Here's the drawing with two shaded views (mm, measured from the low corner). I have some questions. Give positions to 0.01 mm unless a question says otherwise; leave off trailing zeros. Loops run counter-clockwise (first coordinate to the right, second up) from the corner with the lowest first, then second, coordinate; pieces in that order, holes last. Notation, with made-up numbers: M 28.25,78 L 63.25,78 A27 cw 63.25,113 Z; hole C -5,-33 d8. An arc over 180 degrees is marked long. Put each result on its own line as item: value. Start each with the question number.
1) Imagine slicing it at A-A (z = 10). Write out the boundary of the cut face in (x, y).
2) Imagine slicing it at B-B (z = 18.25). Write out the boundary of the cut face in (x, y).
3) If we mould it in two halves opening along X, with no side actions, what happens to the marked faces 1, 2 and 3? For each: +X half, -X half, draft (parallel to the pull), parting line (faces both ways), or undercut.
4) For P1, Ø1.5, axis at x = 4.5, y = 5.5, coming from the -Z side, with a flat end and sliding along its axis, tell me the tip position at first contact or that it passes through.
5) Please list where these lines run through material, in increasing order: line 1 along Z through (x, y) = (3, 2); line 2 along X through (y, z) = (4.8, 10); line 3 along Z through (x, y) = (1.75, 4) (1 decimal). Write a range as from..to.
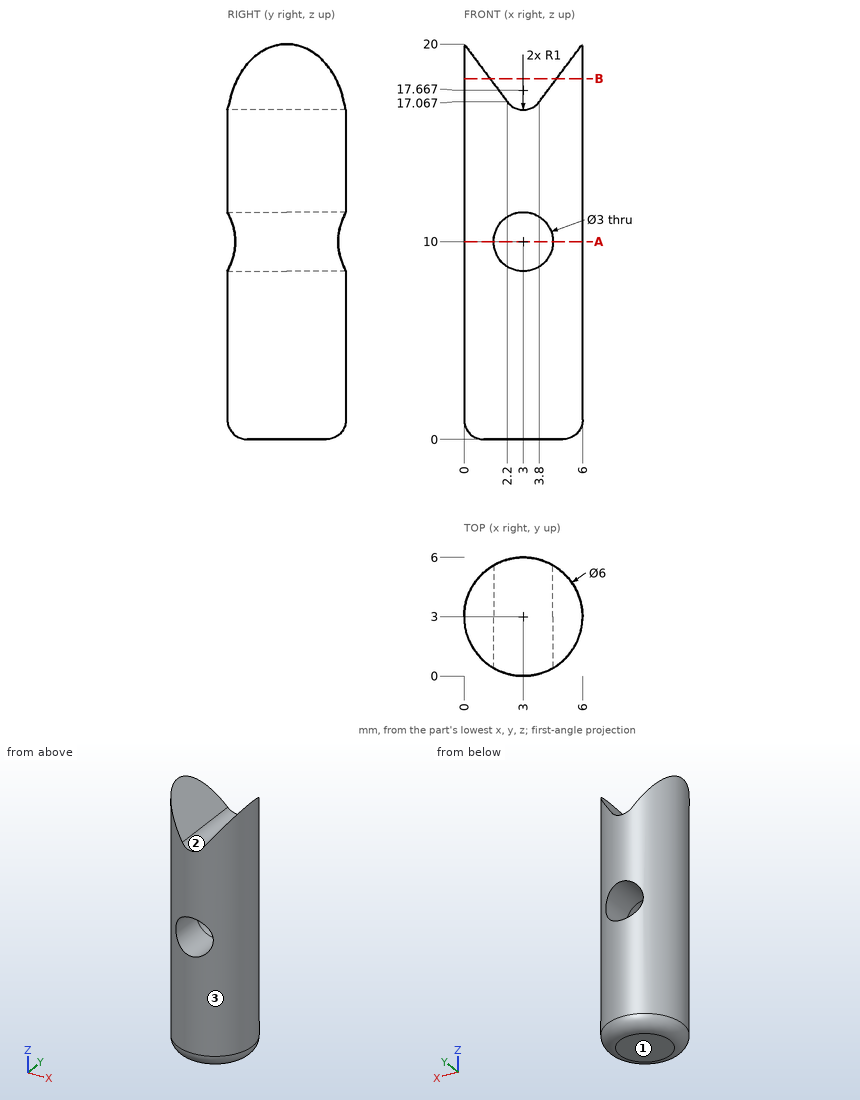
Recorded:
1. outline: M 1.5,0.4 L 1.5,5.6 A3 ccw Z; M 4.5,0.4 A3 ccw 4.5,5.6 Z
2. outline: M 1.31,0.52 L 1.31,5.48 A3 ccw Z; M 4.69,0.52 A3 ccw 4.69,5.48 Z
3. face 1: draft
3. face 2: undercut
3. face 3: parting line
4. P1: z = 0.01
5. line 1: 0..8.5, 11.5..16.67
5. line 2: 0.6..1.5, 4.5..5.4
5. line 3: 0..9.2, 10.8..17.7
